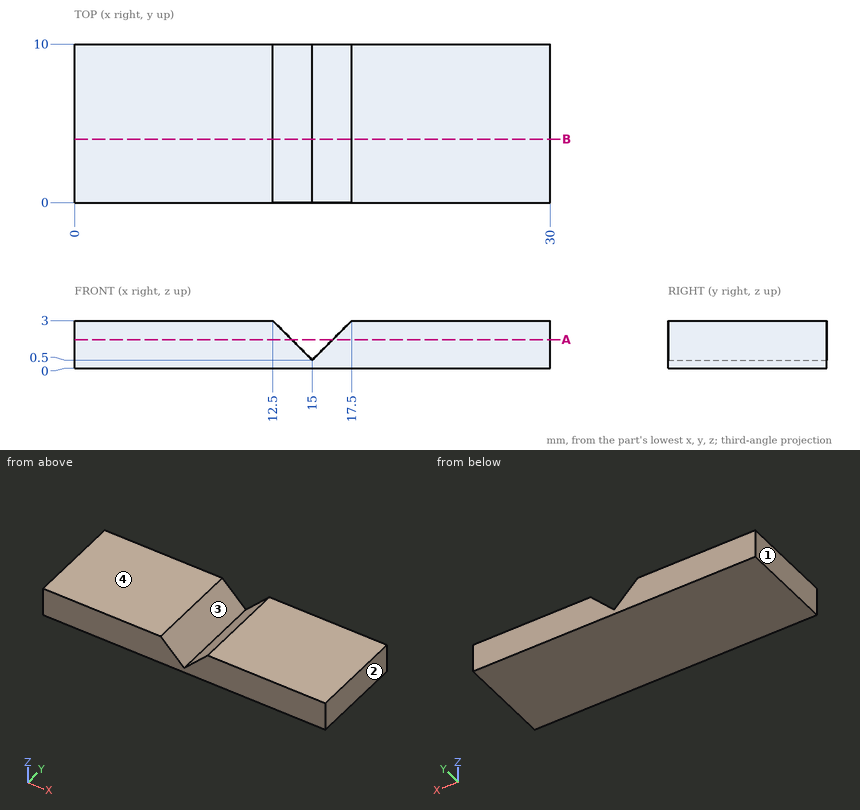
Design review of the part shown in the three views and the two pictorial views. Dimensions are in mm from the part's minimum x, y and z. Give positions to 0.01 mm unless a question says otherwise; leave off trailing zeros. Loops run counter-clockwise (first coordinate to the right, second up) from the corner with the lowest first, then second, coordinate; pieces in that order, holes last. Notation, with made-up numbers: (70.25, 24) -> (114.25, 24) arc R27 ccw to (114.25, 58) -> close; hole circle Ø6 at (-8, 75). An arc over 180 degrees is marked (long way). Answer as a JSON object with one key per item and string values. Group by question number.
Q1. Take a section at B-B (y = 4). Write out the cut boundary in (x, z).
Q2. Draft analysis for pull direction X (two halves, no side actions). For the marked faces 1, 2, 3 and 4, state which applies: pulls with the +X half, pulls with the -X half, needs draft (parallel to the pull), parting line crosses it, or undercut.
Q3. Wall thickness on line 1 along X through (y, z) = (0.5, 0.75); line 2 along X through (y, z) = (6.25, 2.1); line 3 along Z through (x, y) = (14.25, 9.25): over which ranges is each line inside the solid? List them lowest first.
Q4. Take a section at A-A (z = 1.8). Write out the cut boundary in (x, y).
Answer below:
{
 "1": {"outline": "(0, 0) -> (30, 0) -> (30, 3) -> (17.5, 3) -> (15, 0.5) -> (12.5, 3) -> (0, 3) -> close"},
 "2": {"face 1": "pulls with the -X half", "face 2": "pulls with the +X half", "face 3": "undercut", "face 4": "needs draft"},
 "3": {"line 1": "x = 0 to 14.75, 15.25 to 30", "line 2": "x = 0 to 13.4, 16.6 to 30", "line 3": "z = 0 to 1.25"},
 "4": {"outline": "(0, 0) -> (13.7, 0) -> (13.7, 10) -> (0, 10) -> close; (16.3, 0) -> (30, 0) -> (30, 10) -> (16.3, 10) -> close"}
}
